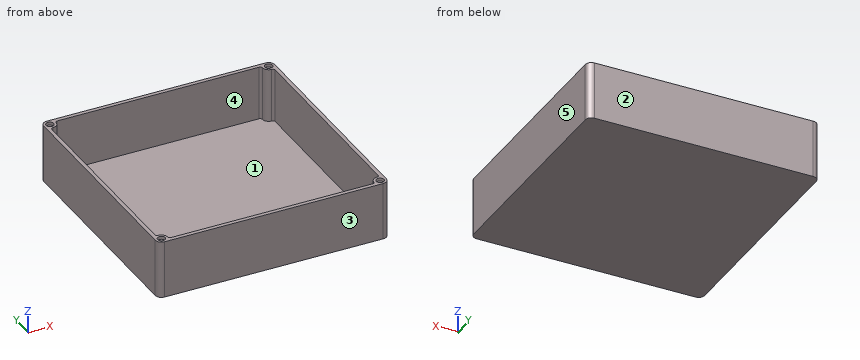
Autodesk Inventor part; units mm, degrees
ref_plane "YZ Plane" through (0, 0, 0) normal (1, 0, 0) x (0, 1, 0)
ref_plane "XZ Plane" through (0, 0, 0) normal (0, 1, 0) x (-1, 0, 0)
ref_plane "XY Plane" through (0, 0, 0) normal (0, 0, 1) x (1, 0, 0)
sketch "Sketch1" plane through (0, 0, 0) normal (0, 0, 1) x (1, 0, 0)
  line L0 (-75, -75) -> (75, -75)
  line L1 (75, -75) -> (75, 75)
  line L2 (75, 75) -> (-75, 75)
  line L3 (-75, 75) -> (-75, -75)
  line L4 (-75, -75) -> (75, 75) construction
  line L5 (75, -75) -> (-75, 75) construction
  line L6 (72.5, -72.5) -> (-72.5, -72.5)
  line L7 (-72.5, -72.5) -> (-72.5, 72.5)
  line L8 (-72.5, 72.5) -> (72.5, 72.5)
  line L9 (72.5, 72.5) -> (72.5, -72.5)
  line L10 (72.5, -72.5) -> (-72.5, 72.5) construction
  line L11 (-72.5, -72.5) -> (72.5, 72.5) construction
  line L12 (-75, 75) -> (-71, 75) construction
  line L13 (-71, 75) -> (-71, 71) construction
  line L14 (-71, 71) -> (-75, 71) construction
  line L15 (-75, 71) -> (-75, 75) construction
  circle A0 centre (-71, 71) radius 2.5
  line L16 (-71, -71) -> (-71, -75) construction
  line L17 (-75, -71) -> (-71, -71) construction
  circle A1 centre (-71, -71) radius 2.5
  line L18 (72.5, 72.5) -> (-72.5, -72.5) construction
  line L19 (75, 75) -> (-75, -75) construction
  line L20 (71, -71) -> (75, -71) construction
  line L21 (71, -75) -> (71, -71) construction
  circle A2 centre (71, -71) radius 2.5
  line L22 (-72.5, 72.5) -> (72.5, -72.5) construction
  line L23 (-75, 75) -> (75, -75) construction
  line L24 (71, 71) -> (71, 75) construction
  line L25 (75, 71) -> (71, 71) construction
  circle A3 centre (71, 71) radius 2.5
  line L26 (-72.5, -72.5) -> (72.5, 72.5) construction
  line L27 (-75, -75) -> (75, 75) construction
  line L28 (-73.5, 73.5) -> (-68.5, 73.5)
  line L29 (-68.5, 73.5) -> (-68.5, 68.5)
  line L30 (-68.5, 68.5) -> (-73.5, 68.5)
  line L31 (-73.5, 68.5) -> (-73.5, 73.5)
  line L32 (-73.5, 73.5) -> (-68.5, 68.5) construction
  line L33 (-68.5, 73.5) -> (-73.5, 68.5) construction
  line L34 (-72.5, -72.5) -> (72.5, 72.5) construction
  line L35 (72.5, 72.5) -> (-72.5, -72.5) construction
  line L36 (-75, -75) -> (75, 75) construction
  line L37 (75, 75) -> (-75, -75) construction
  line L38 (-73.5, -68.5) -> (-68.5, -68.5)
  line L39 (-73.5, -73.5) -> (-68.5, -68.5) construction
  line L40 (-68.5, -68.5) -> (-68.5, -73.5)
  line L41 (-68.5, -73.5) -> (-73.5, -73.5)
  line L42 (-73.5, -73.5) -> (-73.5, -68.5)
  line L43 (72.5, -72.5) -> (-72.5, 72.5) construction
  line L44 (-72.5, 72.5) -> (72.5, -72.5) construction
  line L45 (75, -75) -> (-75, 75) construction
  line L46 (-75, 75) -> (75, -75) construction
  line L47 (68.5, -73.5) -> (68.5, -68.5)
  line L48 (73.5, -73.5) -> (68.5, -68.5) construction
  line L49 (68.5, -68.5) -> (73.5, -68.5)
  line L50 (73.5, -68.5) -> (73.5, -73.5)
  line L51 (73.5, -73.5) -> (68.5, -73.5)
  line L52 (72.5, 72.5) -> (-72.5, -72.5) construction
  line L53 (-72.5, -72.5) -> (72.5, 72.5) construction
  line L54 (75, 75) -> (-75, -75) construction
  line L55 (-75, -75) -> (75, 75) construction
  line L56 (73.5, 68.5) -> (68.5, 68.5)
  line L57 (73.5, 73.5) -> (68.5, 68.5) construction
  line L58 (68.5, 68.5) -> (68.5, 73.5)
  line L59 (68.5, 73.5) -> (73.5, 73.5)
  line L60 (73.5, 73.5) -> (73.5, 68.5)
  line L61 (-72.5, 68.5) -> (-72.5, 67)
  line L62 (-72.5, 67) -> (-67, 67)
  line L63 (-67, 67) -> (-67, 72.5)
  line L64 (-67, 72.5) -> (-68.5, 72.5)
  line L65 (-68.5, 72.5) -> (-68.5, 68.5)
  line L66 (-68.5, 68.5) -> (-72.5, 68.5)
  line L67 (-67, -67) -> (-72.5, -67)
  line L68 (-67, -72.5) -> (-67, -67)
  line L69 (72.5, 72.5) -> (-72.5, -72.5) construction
  line L70 (72.5, 72.5) -> (-72.5, -72.5) construction
  line L71 (-72.5, -72.5) -> (72.5, 72.5) construction
  line L72 (-72.5, -72.5) -> (72.5, 72.5) construction
  line L73 (-75, -75) -> (75, 75) construction
  line L74 (-75, -75) -> (75, 75) construction
  line L75 (75, 75) -> (-75, -75) construction
  line L76 (75, 75) -> (-75, -75) construction
  line L77 (67, -67) -> (67, -72.5)
  line L78 (72.5, -67) -> (67, -67)
  line L79 (-72.5, 72.5) -> (72.5, -72.5) construction
  line L80 (-72.5, 72.5) -> (72.5, -72.5) construction
  line L81 (72.5, -72.5) -> (-72.5, 72.5) construction
  line L82 (72.5, -72.5) -> (-72.5, 72.5) construction
  line L83 (75, -75) -> (-75, 75) construction
  line L84 (75, -75) -> (-75, 75) construction
  line L85 (-75, 75) -> (75, -75) construction
  line L86 (-75, 75) -> (75, -75) construction
  line L87 (67, 67) -> (72.5, 67)
  line L88 (67, 72.5) -> (67, 67)
  line L89 (-72.5, -72.5) -> (72.5, 72.5) construction
  line L90 (-72.5, -72.5) -> (72.5, 72.5) construction
  line L91 (72.5, 72.5) -> (-72.5, -72.5) construction
  line L92 (72.5, 72.5) -> (-72.5, -72.5) construction
  line L93 (75, 75) -> (-75, -75) construction
  line L94 (75, 75) -> (-75, -75) construction
  line L95 (-75, -75) -> (75, 75) construction
  line L96 (-75, -75) -> (75, 75) construction
  line L97 (-72.5, -67) -> (-72.5, -68.5)
  line L98 (-72.5, -68.5) -> (-68.5, -68.5)
  line L99 (-68.5, -68.5) -> (-68.5, -72.5)
  line L100 (-68.5, -72.5) -> (-67, -72.5)
  line L101 (-67, -72.5) -> (-67, -67)
  line L102 (-67, -67) -> (-72.5, -67)
  line L103 (68.5, -72.5) -> (67, -72.5)
  line L104 (67, -72.5) -> (67, -67)
  line L105 (67, -67) -> (72.5, -67)
  line L106 (72.5, -67) -> (72.5, -68.5)
  line L107 (72.5, -68.5) -> (68.5, -68.5)
  line L108 (68.5, -68.5) -> (68.5, -72.5)
  line L109 (67, 72.5) -> (68.5, 72.5)
  line L110 (68.5, 72.5) -> (68.5, 68.5)
  line L111 (68.5, 68.5) -> (72.5, 68.5)
  line L112 (72.5, 68.5) -> (72.5, 67)
  line L113 (72.5, 67) -> (67, 67)
  line L114 (67, 67) -> (67, 72.5)
  point P0 (0, 0)
  point P1 (0, 0)
  point P2 (0, 0)
  point P3 (0, 0)
  point P4 (0, 0)
  point P5 (0, 0)
  point P6 (0, 0)
  point P7 (0, 0)
  point P8 (0, 0)
  point P9 (0, 0)
  point P10 (0, 0)
  point P11 (0, 0)
  point P12 (0, 0)
  point P13 (0, 0)
  point P14 (0, 0)
  point P15 (0, 0)
  point P16 (0, 0)
  point P17 (0, 0)
  point P18 (-68.5, 68.5)
  point P19 (0, 0)
  point P20 (0, 0)
  point P21 (0, 0)
  point P22 (0, 0)
  point P23 (-68.5, -68.5)
  dimension "d0" = 150
  dimension "d1" = 150
  dimension "d2" = 145
  dimension "d3" = 145
  dimension "d8" = 4
  dimension "d9" = 4
  dimension "d10" = 5
  dimension "d13" = 360
  dimension "d17" = 360
  dimension "d25" = 1.5
  dimension "d28" = 360
extrude "Extrusion1" add sketch "Sketch1" along normal blind 2.5 contours L47 A2 L6 | L6 L77 L78 L9 L49 L47 | L6 L68 L67 L7 L62 L63 L8 L88 L87 L9 L78 L77 | A2 L9 L6 | L47 L49 A2 | L6 L40 L38 L7 L67 L68 | L49 L9 A2 | L6 A1 L40 | L6 L7 A1 | A1 L38 L40 | L87 L88 L8 L58 L56 L9 | A1 L7 L38 | L7 L30 L29 L8 L63 L62 | L56 A3 L9 | L7 A0 L30 | A3 L8 L9 | L56 L58 A3 | L7 L8 A0 | A0 L29 L30 | L58 L8 A3 | A0 L8 L29 picked at (70.3289, -70.3289) picked at (-70.3289, -70.3289) picked at (70.3289, 70.3289) picked at (-70.3289, 70.3289)
extrude "Extrusion2" add sketch "Sketch1" along normal blind 37.5 contours L3 L2 L1 L0 | L6 A2 L51 L47 | L6 L9 A2 | A2 L50 L51 | L40 L41 A1 L6 | L9 L49 L50 A2 | A1 L7 L6 | L41 L42 A1 | L7 A1 L42 L38 | L9 A3 L60 L56 | L30 L31 A0 L7 | L9 L8 A3 | A0 L8 L7 | A3 L59 L60 | L58 L59 A3 L8 | L31 L28 A0 | L8 A0 L28 L29 picked at (72.6398, -70.2994) picked at (-72.6398, -70.2994) picked at (72.6398, 70.2994) picked at (-72.6398, 70.2994)
extrude "Extrusion3" add sketch "Sketch1" along normal blind 37.5 contours L47 A2 L6 | L6 A2 L51 L47 | A2 L9 L6 | L6 L9 A2 | L47 L49 A2 | A2 L50 L51 | L49 L9 A2 | L40 L41 A1 L6 | L6 A1 L40 | L9 L49 L50 A2 | A1 L7 L6 | L6 L7 A1 | A1 L38 L40 | L41 L42 A1 | A1 L7 L38 | L7 A1 L42 L38 | L56 A3 L9 | L9 A3 L60 L56 | L30 L31 A0 L7 | L7 A0 L30 | A3 L8 L9 | L9 L8 A3 | L56 L58 A3 | A0 L8 L7 | L7 L8 A0 | A0 L29 L30 | A3 L59 L60 | L58 L8 A3 | L58 L59 A3 L8 | L31 L28 A0 | A0 L8 L29 | L8 A0 L28 L29
extrude "Extrusion4" cut sketch "Sketch1" along normal blind 37.5 contours A2 L9 L6 | L6 L9 A2 | A1 L7 L6 | L6 L7 A1 | A3 L8 L9 | L9 L8 A3 | A0 L8 L7 | L7 L8 A0
extrude "Extrusion5" add sketch "Sketch1" along normal blind 35.5 contours A2 L9 L6 | L6 L9 A2 | A1 L7 L6 | L6 L7 A1 | A3 L8 L9 | L9 L8 A3 | A0 L8 L7 | L7 L8 A0
extrude "Extrusion6" add sketch "Sketch1" along normal blind 37.5 contours L47 A2 L6 | L6 A2 L51 L47 | L6 L77 L78 L9 L49 L47 | L6 L68 L67 L7 L62 L63 L8 L88 L87 L9 L78 L77 | A2 L9 L6 | L6 L9 A2 | L47 L49 A2 | L6 L40 L38 L7 L67 L68 | A2 L50 L51 | L49 L9 A2 | L40 L41 A1 L6 | L6 A1 L40 | L9 L49 L50 A2 | A1 L7 L6 | L6 L7 A1 | A1 L38 L40 | L87 L88 L8 L58 L56 L9 | L41 L42 A1 | A1 L7 L38 | L7 A1 L42 L38 | L7 L30 L29 L8 L63 L62 | L56 A3 L9 | L9 A3 L60 L56 | L30 L31 A0 L7 | L7 A0 L30 | A3 L8 L9 | L9 L8 A3 | L56 L58 A3 | A0 L8 L7 | L7 L8 A0 | A0 L29 L30 | A3 L59 L60 | L58 L8 A3 | L58 L59 A3 L8 | L31 L28 A0 | A0 L8 L29 | L8 A0 L28 L29
extrude "Extrusion7" cut sketch "Sketch1" along normal blind 37.5 contours L6 L68 L67 L7 L62 L63 L8 L88 L87 L9 L78 L77 | A2 L9 L6 | L6 L9 A2 | A1 L7 L6 | L6 L7 A1 | A3 L8 L9 | L9 L8 A3 | A0 L8 L7 | L7 L8 A0
extrude "Extrusion8" add sketch "Sketch1" along normal blind 2.5 contours L47 A2 L6 | L6 A2 L51 L47 | L6 L77 L78 L9 L49 L47 | L6 L68 L67 L7 L62 L63 L8 L88 L87 L9 L78 L77 | A2 L9 L6 | L6 L9 A2 | L47 L49 A2 | L6 L40 L38 L7 L67 L68 | A2 L50 L51 | L49 L9 A2 | L40 L41 A1 L6 | L6 A1 L40 | L9 L49 L50 A2 | A1 L7 L6 | L6 L7 A1 | A1 L38 L40 | L87 L88 L8 L58 L56 L9 | L41 L42 A1 | A1 L7 L38 | L7 A1 L42 L38 | L7 L30 L29 L8 L63 L62 | L56 A3 L9 | L9 A3 L60 L56 | L30 L31 A0 L7 | L7 A0 L30 | A3 L8 L9 | L9 L8 A3 | L56 L58 A3 | A0 L8 L7 | L7 L8 A0 | A0 L29 L30 | A3 L59 L60 | L58 L8 A3 | L58 L59 A3 L8 | L31 L28 A0 | A0 L8 L29 | L8 A0 L28 L29
extrude "Extrusion9" add sketch "Sketch1" along normal blind 35.5 contours A2 L9 L6 | L6 L9 A2 | A1 L7 L6 | L6 L7 A1 | A3 L8 L9 | L9 L8 A3 | A0 L8 L7 | L7 L8 A0
fillet "Fillet1" radius 4 4 edges at (-75, -75, 18.75) (75, -75, 18.75) (75, 75, 18.75) (-75, 75, 18.75)
fillet "Fillet2" radius 4 4 edges at (-67, 67, 20) (-67, -67, 20) (67, 67, 20) (67, -67, 20)
fillet "Fillet3" radius 1.5 8 edges at (-67, 72.5, 20) (-72.5, 67, 20) (67, 72.5, 20) (72.5, 67, 20) (67, -72.5, 20) (72.5, -67, 20) (-72.5, -67, 20) (-67, -72.5, 20)
properties part number "electronics_box_small"
CAD build for the part. Positions are in the model's coordinates, mm. Face numbers are marked on the shaded views. A direction names the side the tool comes from. Coordinates: 2 decimals unless noted, no trailing zeros. Order: outer loops, then holes, each group sorted by start corner. A loop starts at its lowest first (then second) coordinate and runs counter-clockwise, first axis right, second up. Notation, with made-up numbers: (19.25, -8) - (23.25, -8) arc R29 cw to (23.25, 23) - close; hole circle Ø11 at (31.25, 9.25). An arc over 180 degrees is marked (long way). Answer in a Markdown table with one row per item.
1. 3-axis set-ups, long thin cutter, end or side, ignore diameter. For the marked faces 1 and 2: which of +Z, -Z, +X, -X, +Y, -Y reach the whole face in a straight line?
Answer:
| item | result |
|---|---|
| face 1 | +Z |
| face 2 | +Z, -Z, +X, -X, +Y |
2. Slice it at B-B, the plane x = 48. List the corners of the cut face in (y, z), then the cut area to 3 significant figures.
Answer:
| item | result |
|---|---|
| outline | (-75, 0) - (75, 0) - (75, 37.5) - (72.5, 37.5) - (72.5, 2.5) - (-72.5, 2.5) - (-72.5, 37.5) - (-75, 37.5) - close |
| area | 550 mm² |
3. Flat gauge pins, fed straight in: P1, Ø8, axis at x = -71, y = -71, coming from the -Z side; P2, Ø3, axis at x = 71, y = -71, coming from the +Z side; P3, Ø5, axis at x = -52, y = -30.5, coming from the +Z side. Where does each tip first touch, or does it go through?
Answer:
| item | result |
|---|---|
| P1 | z = 0 |
| P2 | z = 35.5 |
| P3 | z = 2.5 |
4. Drill centre lines: L1, parallel to X at y = 71, z = 36; L2, parallel to X at y = -0.5, z = 4.5. Where is each one in solid material? Low to high. Write a range as from..to.
Answer:
| item | result |
|---|---|
| L1 | -75..-73.5, -68.5..-67, 67..68.5, 73.5..75 |
| L2 | -75..-72.5, 72.5..75 |
5. Pull direction Y, two halves, no side cores. Call the marked faces 3, 4 and 5: +Y half, -Y half, draft (parallel to the pull), parting line (faces both ways), or undercut.
Answer:
| item | result |
|---|---|
| face 3 | -Y half |
| face 4 | undercut |
| face 5 | draft |
